Study the drawing (mm; zero at the part's minimum x, y, z) and answer. Coordinates: 2 decimals unless noted, no trailing zeros. Order: outer loops, then holes, each group sorted by start corner. A loop starts at its lowest first (then second) coordinate and runs counter-clockwise, first axis right, second up.
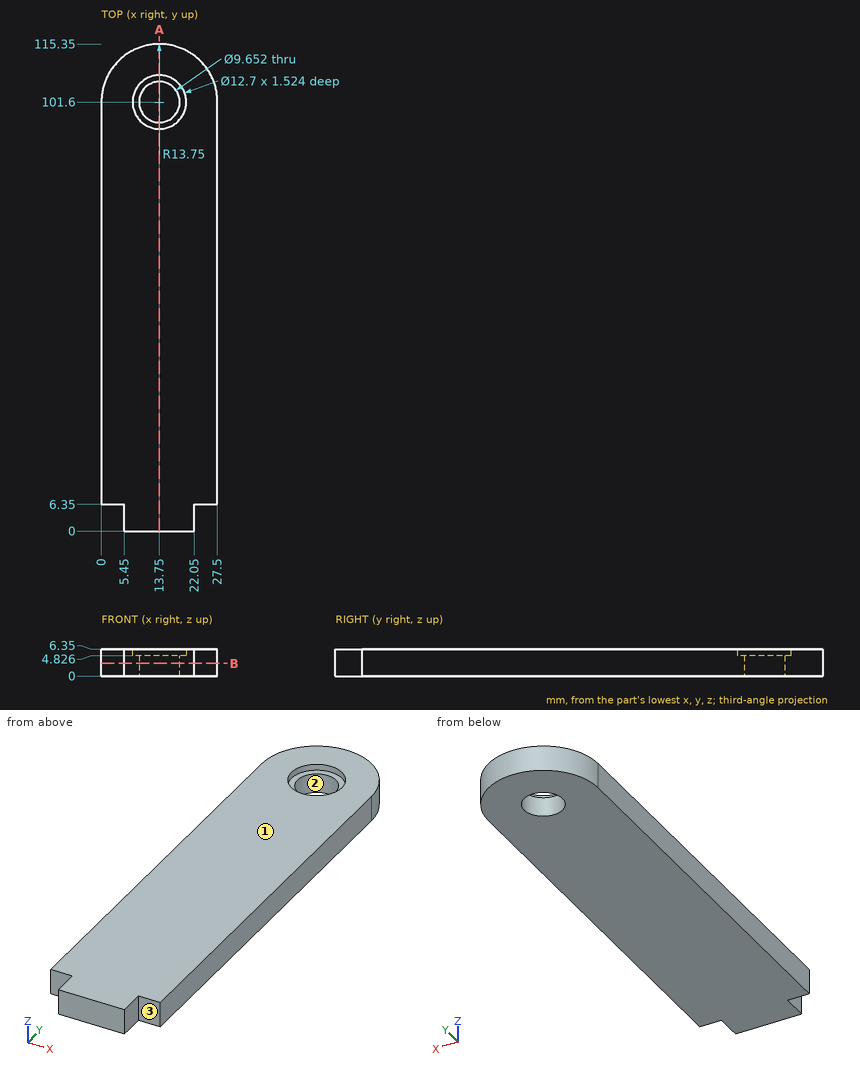
1) A cutting plane is placed at A-A, the plane x = 13.75. Determine the outline of the cut face in (y, z).
A:
outline: (0, 0) - (96.77, 0) - (96.77, 4.83) - (95.25, 4.83) - (95.25, 6.35) - (0, 6.35) - close; (106.43, 0) - (115.35, 0) - (115.35, 6.35) - (107.95, 6.35) - (107.95, 4.83) - (106.43, 4.83) - close
2) Straight lines are drawn through the part: line 1 (Y direction, x = 13.75, z = 5.75); line 2 (Y direction, x = 13.75, z = 1); line 3 (X direction, y = 109, z = 2.25). For each, find the intervals that lie inside material, in ascending order.
A:
line 1: y = 0 to 95.25, 107.95 to 115.35
line 2: y = 0 to 96.77, 106.43 to 115.35
line 3: x = 2.16 to 25.34
3) Determine the mould class of the marked faces 1, 2 and 3 for opening direction Y: pulls with the +Y half, pulls with the -Y half, needs draft (parallel to the pull), parting line crosses it, or undercut.
A:
face 1: needs draft
face 2: undercut
face 3: pulls with the -Y half
4) Flat-ended cylindrical pins translate along their axes: pin 1 Ø2.5 at (x, z) = (1.5, 2.5) entering from -Y; pin 2 Ø1.9 at (y, z) = (2.5, 3.5) entering from -X; pin 3 Ø8.5 at (x, y) = (13.75, 101.6) entering from -Z. Find the tip coordinate at first contact, or state that the pin passes through.
A:
pin 1: stops at y = 6.35
pin 2: stops at x = 5.45
pin 3: passes through
5) A cutting plane is placed at B-B, the plane z = 3. Determine the outline of the cut face in (x, y).
A:
outline: (0, 6.35) - (5.45, 6.35) - (5.45, 0) - (22.05, 0) - (22.05, 6.35) - (27.5, 6.35) - (27.5, 101.6) arc R13.75 ccw to (0, 101.6) - close; hole circle Ø9.65 at (13.75, 101.6)
